Can you work these out from the drawing? Everything is in mm from the part's minimum corner. Coordinates: 2 decimals unless noted, no trailing zeros. Loops run counter-clockwise (first coordinate to the right, second up) from the corner with the lowest first, then second, coordinate; pieces in that order, holes last. Notation, with made-up numbers: M 79.5,-24.5 L 84.5,-24.5 A32 ccw 84.5,4.5 Z; hole C 42.5,1.5 d5. An arc over 180 degrees is marked long. Use CSV: the item, a comma, the result in double quotes. Start each with the question number.
Q1. For pin 1 Ø12 at (x, z) = (102, 13.5) entering from -Y; pin 2 Ø3 at (y, z) = (5, 40.5) entering from -X; pin 3 Ø1 at (x, z) = (34, 54.5) entering from +Y; pin 4 Ø3 at (y, z) = (6.5, 56) entering from -X, each with a flat end and sliding along its axis, tell me the tip position at first contact or that it passes through.
Q2. If we mould it in two halves opening along X, with no side actions, what happens to the marked faces 1 and 2? For each: +X half, -X half, draft (parallel to the pull), parting line (faces both ways), or undercut.
Q3. If we section it at C-C (y = 9.5): Please give me the cut outline in (x, z) (1 decimal).
Q4. If we section it at A-A (z = 48): Please give me the cut outline in (x, y).
Q5. Please list where these lines run through material, in increasing order: probe 1 along X at (y, z) = (7.5, 3.5); probe 2 along Z at (x, y) = (143.5, 4.25); probe 3 along X at (y, z) = (8.25, 59.5). Write a range as [from, to].
Q6. If we section it at D-D (z = 3.5): Please give me the cut outline in (x, y).
Q7. If we section it at B-B (x = 13): Please give me the cut outline in (y, z).
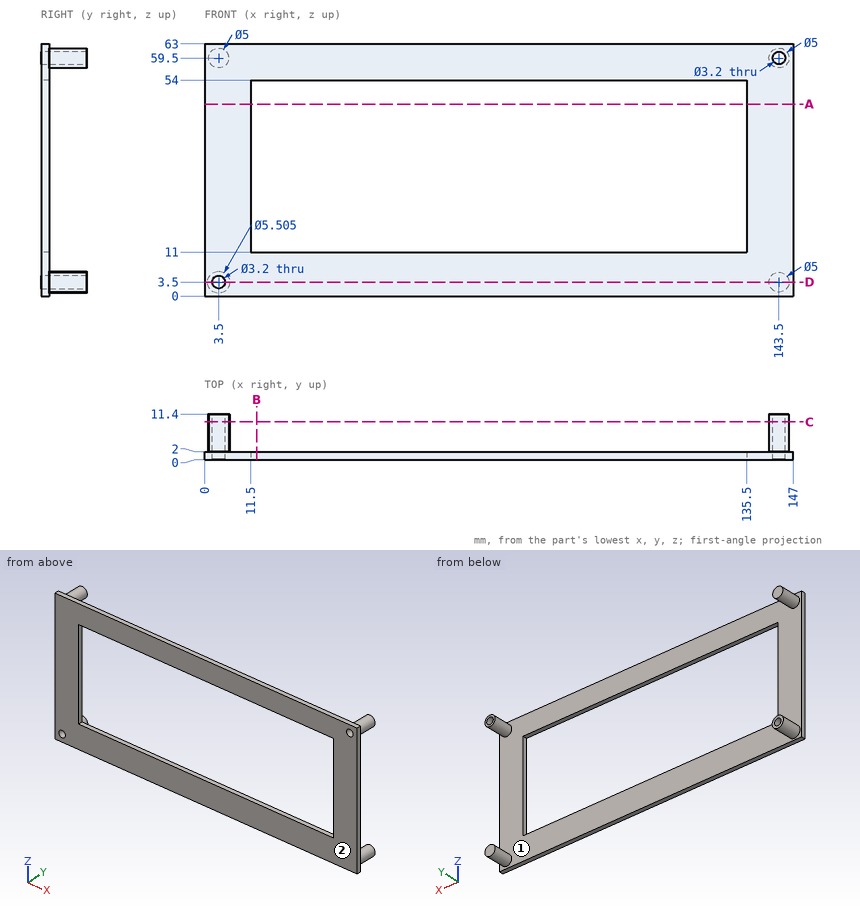
Results below:
1,pin 1,"y = 0"
1,pin 2,"through"
1,pin 3,"y = 2"
1,pin 4,"x = 2"
2,face 1,"undercut"
2,face 2,"draft"
3,outline,"C 3.5,3.5 d5.5; C 3.5,59.5 d5; C 143.5,3.5 d5; C 143.5,59.5 d5; hole C 3.5,3.5 d3.2; hole C 143.5,59.5 d3.2"
4,outline,"M 0,0 L 11.5,0 L 11.5,2 L 0,2 Z; M 135.5,0 L 147,0 L 147,2 L 135.5,2 Z"
5,probe 1,"[0.75, 1.9], [5.1, 6.25], [141, 146]"
5,probe 2,"[1, 6], [57, 57.9], [61.1, 62]"
5,probe 3,"[1, 6], [141, 141.9], [145.1, 146]"
6,outline,"M 0,0 L 1.9,0 L 1.9,11.4 L 0.75,11.4 L 0.75,2 L 0,2 Z; M 5.1,0 L 147,0 L 147,2 L 146,2 L 146,11.4 L 141,11.4 L 141,2 L 6.25,2 L 6.25,11.4 L 5.1,11.4 Z"
7,outline,"M 0,0 L 2,0 L 2,11 L 0,11 Z; M 0,54 L 2,54 L 2,63 L 0,63 Z"
